Can you work these out from the drawing? Everything is in mm from the part's minimum corner. A direction names the side the tool comes from. Coordinates: 2 decimals unless noted, no trailing zeros. Order: outer loops, then holes, each group sorted by start corner. A loop starts at its lowest first (then second) coordinate and runs counter-clockwise, first axis right, second up. Notation, with made-up numbers: (48.5, 41.5) - (66.5, 41.5) arc R23 ccw to (66.5, 55.5) - close; hole circle Ø9 at (41, 84.25). An arc over 180 degrees is marked (long way). One line per item, written item: value.
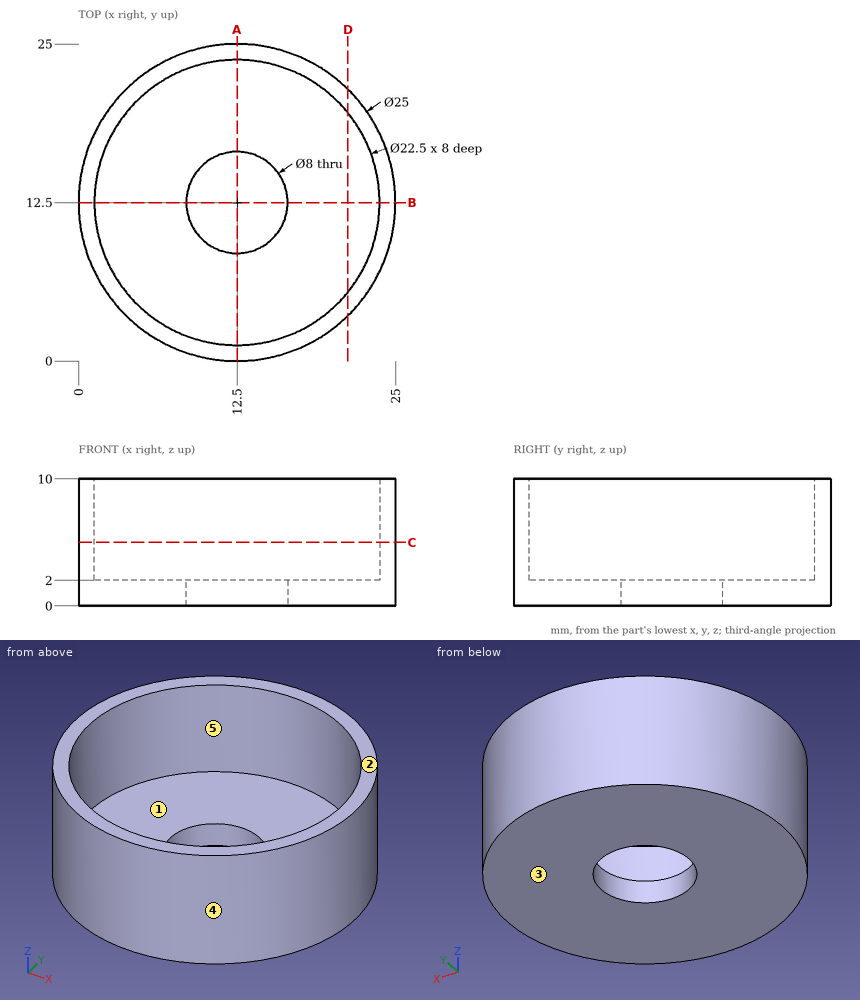
Item 1: I want a section at A-A on x = 12.5. Please give me the cut outline in (y, z).
Conclusion:
outline: (0, 0) - (8.5, 0) - (8.5, 2) - (1.25, 2) - (1.25, 10) - (0, 10) - close; (16.5, 0) - (25, 0) - (25, 10) - (23.75, 10) - (23.75, 2) - (16.5, 2) - close
Item 2: For the marked faces 1 and 2, which set-ups out of +Z, -Z, +X, -X, +Y, -Y let a thin tool reach every point of the face, with its end or its side?
Conclusion:
face 1: +Z
face 2: +Z, +X, -X, +Y, -Y
Item 3: I want a section at D-D on x = 21.25. Please give me the cut outline in (y, z).
Conclusion:
outline: (3.57, 0) - (21.43, 0) - (21.43, 10) - (19.57, 10) - (19.57, 2) - (5.43, 2) - (5.43, 10) - (3.57, 10) - close
Item 4: If I drill on probe 1 along Y at (x, z) = (12.5, 8.25); probe 2 along Y at (x, z) = (12.5, 1.3); probe 3 along Z at (x, y) = (16, 14.5), over which ranges is the centre line in solid material (lowest first)?
Conclusion:
probe 1: 0 to 1.25, 23.75 to 25
probe 2: 0 to 8.5, 16.5 to 25
probe 3: 0 to 2
Item 5: I want a section at C-C on z = 5. Please give me the cut outline in (x, y), then the cut area to 3 significant figures.
Conclusion:
outline: circle Ø25 at (12.5, 12.5); hole circle Ø22.5 at (12.5, 12.5)
area: 93.3 mm²
Item 6: Thinking about a two-plate mould opening in X: for the marked faces 3, 4 and 5, which applies, pulls with the +X half, pulls with the -X half, needs draft (parallel to the pull), parting line crosses it, or undercut?
Conclusion:
face 3: needs draft
face 4: parting line crosses it
face 5: undercut
Item 7: I'm going to push flat-ended pins straight in: pin 1 Ø3 at (y, z) = (19, 6.5) entering from -X; pin 2 Ø4 at (y, z) = (17, 2.5) entering from +X; pin 3 Ø13.5 at (x, y) = (12.5, 12.5) entering from +Z. Where does each tip first touch, or does it pass through?
Conclusion:
pin 1: x = 1.04
pin 2: x = 24.75
pin 3: z = 2
